Verification items for this drawing (mm, ordinates from the low corner). A direction names the side the tool comes from. Round coordinates to 2 decimals unless told otherwise and drop trailing zeros. Loops run counter-clockwise (first coordinate to the right, second up) from the corner with the lowest first, then second, coordinate; pieces in that order, holes last. Notation, with made-up numbers: (8, 17) - (63, 17) arc R25 ccw to (63, 46) - close; hole circle Ø6 at (32.5, -11). An arc over 180 degrees is marked (long way). Answer in a Markdown table with one row per item. Add a question column.
(1) Gauge pin test, flat ends, axial feed: pin 1 (0.8 mm diameter, centred on x = 78.5, y = 11.5, fed in from -Z); pin 2 (10 mm diameter, centred on x = 16, y = 10, fed in from -Z); pin 3 (3 mm diameter, centred on x = 2.5, y = 11.5, fed in from -Z); pin 4 (8 mm diameter, centred on x = 25.5, z = 21, fed in from -Y). Record the tip position at first contact, or that the pin passes through.
(2) Mould release check, pull along X, two halves, no side actions. Record for the marked faces 3, 4 and 5: +X half, -X half, draft (parallel to the pull), parting line (faces both ways), or undercut.
(3) Cross-section at B-B on y = 20. Enter the section's corners in (x, z).
(4) Cross-section at C-C on x = 3. Enter the section's corners in (y, z).
(5) Cross-section at A-A on z = 6.5. Enter the section's corners in (x, y).
(6) Cross-section at D-D on y = 9. Enter the section's corners in (x, z).
(7) Thickness scan on line 1 along Y through (x, z) = (3, 8); line 2 along X through (y, z) = (15.25, 18); line 3 along X through (y, z) = (12.25, 9.5). Record the ranges inside material, lowest first.
(8) Access from +Z, -Z, +X, -X, +Y, -Y to the whole of each face (thin tool, end or side, straight path). Record for the marked faces 1 and 2.
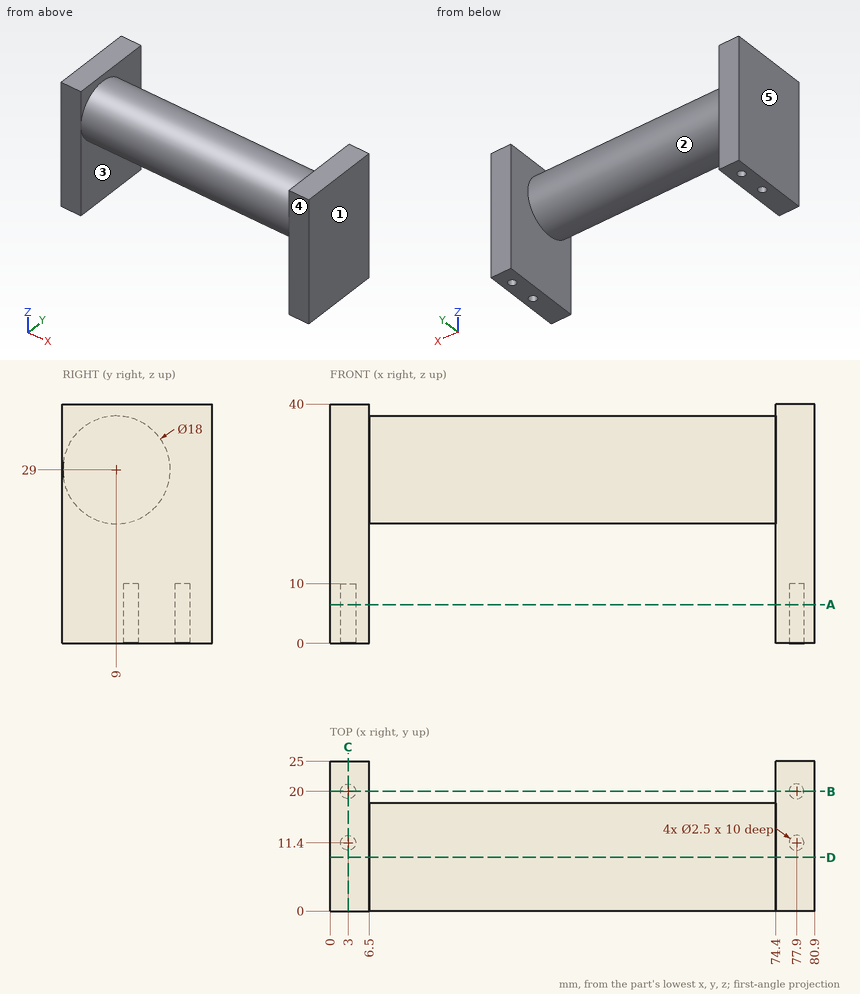
Answers:
| question | item | result |
|---|---|---|
| 1 | pin 1 | stops at z = 10 |
| 1 | pin 2 | stops at z = 20 |
| 1 | pin 3 | stops at z = 0 |
| 1 | pin 4 | stops at y = 0.94 |
| 2 | face 3 | undercut |
| 2 | face 4 | draft |
| 2 | face 5 | -X half |
| 3 | outline | (0, 0) - (1.75, 0) - (1.75, 10) - (4.25, 10) - (4.25, 0) - (6.5, 0) - (6.5, 40) - (0, 40) - close; (74.4, 0) - (76.65, 0) - (76.65, 10) - (79.15, 10) - (79.15, 0) - (80.9, 0) - (80.9, 40) - (74.4, 40) - close |
| 4 | outline | (0, 0) - (10.15, 0) - (10.15, 10) - (12.65, 10) - (12.65, 0) - (18.75, 0) - (18.75, 10) - (21.25, 10) - (21.25, 0) - (25, 0) - (25, 40) - (0, 40) - close |
| 5 | outline | (0, 0) - (6.5, 0) - (6.5, 25) - (0, 25) - close; (74.4, 0) - (80.9, 0) - (80.9, 25) - (74.4, 25) - close; hole circle Ø2.5 at (3, 11.4); hole circle Ø2.5 at (3, 20); hole circle Ø2.5 at (77.9, 11.4); hole circle Ø2.5 at (77.9, 20) |
| 6 | outline | (0, 0) - (6.5, 0) - (6.5, 20) - (74.4, 20) - (74.4, 0) - (80.9, 0) - (80.9, 40) - (74.4, 40) - (74.4, 38) - (6.5, 38) - (6.5, 40) - (0, 40) - close |
| 7 | line 1 | y = 0 to 10.15, 12.65 to 18.75, 21.25 to 25 |
| 7 | line 2 | x = 0 to 6.5, 74.4 to 80.9 |
| 7 | line 3 | x = 0 to 2.08, 3.92 to 6.5, 74.4 to 76.98, 78.82 to 80.9 |
| 8 | face 1 | +Z, -Z, +X, +Y, -Y |
| 8 | face 2 | none |
